from build123d import *

# Parameters (mm, degrees)
F0_R     = 5
F0_R_2   = 2.5
F1_DEPTH = 1
F3_DEPTH = 1


# Not quite as in the source:
# - after a boolean that leaves OpenCascade's solid faulty, fix() repairs it


with BuildPart() as f1:
    # F0 (on Top) → F1 (new body)
    with BuildSketch(Plane.XY):
        Circle(F0_R)
        Circle(F0_R_2, mode=Mode.SUBTRACT)
    extrude(amount=F1_DEPTH)

    # F2 (on face) → F3 (join)
    with BuildSketch(Plane.XY.offset(1)):
        with BuildLine():
            ThreePointArc((-0.4197226159, 2.4645147445), (0, 2.5), (0.4197226159, 2.4645147445))
            Line((0.4197226159, 2.4645147445), (0.4197226159, 4.9823521479))
            Line((0.4197226159, 4.9823521479), (-0.4197226159, 4.9823521479))
            Line((-0.4197226159, 4.9823521479), (-0.4197226159, 2.4645147445))
        make_face()
        with BuildLine():
            ThreePointArc((-2.3441936847, 0.8687669243), (-2.1650635095, 1.25), (-1.9244710687, 1.5957478202))
            Line((-1.9244710687, 1.5957478202), (-4.1049822227, 2.8546665219))
            Line((-4.1049822227, 2.8546665219), (-4.5247048387, 2.127685626))
            Line((-4.5247048387, 2.127685626), (-2.3441936847, 0.8687669243))
        make_face()
        with BuildLine():
            ThreePointArc((-1.9244710687, -1.5957478202), (-2.1650635095, -1.25), (-2.3441936847, -0.8687669243))
            Line((-2.3441936847, -0.8687669243), (-4.5247048387, -2.127685626))
            Line((-4.5247048387, -2.127685626), (-4.1049822227, -2.8546665219))
            Line((-4.1049822227, -2.8546665219), (-1.9244710687, -1.5957478202))
        make_face()
        with BuildLine():
            ThreePointArc((0.4197226159, -2.4645147445), (0, -2.5), (-0.4197226159, -2.4645147445))
            Line((-0.4197226159, -2.4645147445), (-0.4197226159, -4.9823521479))
            Line((-0.4197226159, -4.9823521479), (0.4197226159, -4.9823521479))
            Line((0.4197226159, -4.9823521479), (0.4197226159, -2.4645147445))
        make_face()
        with BuildLine():
            Line((4.5247048387, -2.127685626), (2.3441936847, -0.8687669243))
            ThreePointArc((2.3441936847, -0.8687669243), (2.1650635095, -1.25), (1.9244710687, -1.5957478202))
            Line((1.9244710687, -1.5957478202), (4.1049822227, -2.8546665219))
            Line((4.1049822227, -2.8546665219), (4.5247048387, -2.127685626))
        make_face()
        with BuildLine():
            Line((4.1049822227, 2.8546665219), (1.9244710687, 1.5957478202))
            ThreePointArc((1.9244710687, 1.5957478202), (2.1650635095, 1.25), (2.3441936847, 0.8687669243))
            Line((2.3441936847, 0.8687669243), (4.5247048387, 2.127685626))
            Line((4.5247048387, 2.127685626), (4.1049822227, 2.8546665219))
        make_face()
    extrude(amount=F3_DEPTH)

    add(f1.part.fix(), mode=Mode.REPLACE)


solid = f1.part
Verification items for the finished model (mm, model axes). A direction names the side the tool comes from. Give positions to 0.01 mm unless a question says otherwise; leave off trailing zeros. Write each loop counter-clockwise with the first axis right and the second up, starting at its lowest first coordinate (ties: lowest second). Pieces come first, ordered by that corner, then holes. Notation, with made-up numbers: M 49.25,78 L 88.25,78 A10 cw 88.25,82 Z; hole C 22,-30.75 d1. An arc over 180 degrees is marked long. Use CSV: the item, a comma, the result in double quotes.
1) Cross-section at B-B (z = 1.35). Enter the section's corners in (x, y).
Final values:
outline,"M -4.52,-2.13 L -4.1,-2.85 L -1.92,-1.6 A2.5 cw -2.34,-0.87 Z; M -4.52,2.13 L -2.34,0.87 A2.5 cw -1.92,1.6 L -4.1,2.85 Z; M -0.42,-4.98 L 0.42,-4.98 L 0.42,-2.46 A2.5 cw -0.42,-2.46 Z; M -0.42,2.46 A2.5 cw 0.42,2.46 L 0.42,4.98 L -0.42,4.98 Z; M 1.92,-1.6 L 4.1,-2.85 L 4.52,-2.13 L 2.34,-0.87 A2.5 cw Z; M 1.92,1.6 A2.5 cw 2.34,0.87 L 4.52,2.13 L 4.1,2.85 Z"
2) Cross-section at C-C (x = -1.5). Enter the section's corners in (y, z), plus the area to 3 significant figures.
Final values:
outline,"M -4.77,0 L -2,0 L -2,1 L -4.77,1 Z; M 2,0 L 4.77,0 L 4.77,1 L 2,1 Z"
area,"5.54 mm²"
3) Cross-section at D-D (y = -1.25). Enter the section's corners in (x, z).
Final values:
outline,"M -4.84,0 L -2.17,0 L -2.17,2 L -3,2 L -3,1 L -4.84,1 Z; M 2.17,0 L 4.84,0 L 4.84,1 L 3,1 L 3,2 L 2.17,2 Z"
4) Access from +Z, -Z, +X, -X, +Y, -Y to the whole of each face (thin tool, end or side, straight path). Record for faces 5 (the face through (2, 3, 1)), 6 (the face through (0, 4.982, 1.5)), 7 (the face through (-4, 0, 1)).
Final values:
face 5,"+Z, +Y"
face 6,"+Z, +X, -X, +Y"
face 7,"+Z, -X"
5) Release check for a two-part mould opening along X. For faces 1 (the face through (0, -4, 2)), 2 (the face through (-2, -3, 1)), 3 (the face through (-3.45, 1.507, 1.493)), 4 (the face through (-2.999, 2.216, 1.493)) record: released by +X, released by -X, zero draft, split by the parting line, or undercut.
Final values:
face 1,"zero draft"
face 2,"undercut"
face 3,"released by -X"
face 4,"undercut"
6) Material ranges on line 1 along Y through (x, z) = (0, 0.5); line 2 along Z through (x, y) = (-1, -3.5); line 3 along Y through (x, z) = (-2.5, 1.25), recorded low to high.
Final values:
line 1,"-5 to -2.5, 2.5 to 5"
line 2,"0 to 1"
line 3,"-1.93 to -0.96, 0.96 to 1.93"
7) Go/stop test with flat-tipped pins: pin 1 Ø0.9 at (x, z) = (0, 1.5) entering from +Y; pin 2 Ø1 at (x, y) = (-1, 0.5) entering from -Z; pin 3 Ø1 at (x, y) = (-2, 3) entering from +Z. Record where each tip stops, or that it passes through.
Final values:
pin 1,"y = 4.98"
pin 2,"through"
pin 3,"z = 1"
8) Cross-section at A-A (y = 0). Enter the section's corners in (x, z).
Final values:
outline,"M -5,0 L -2.5,0 L -2.5,1 L -5,1 Z; M 2.5,0 L 5,0 L 5,1 L 2.5,1 Z"
